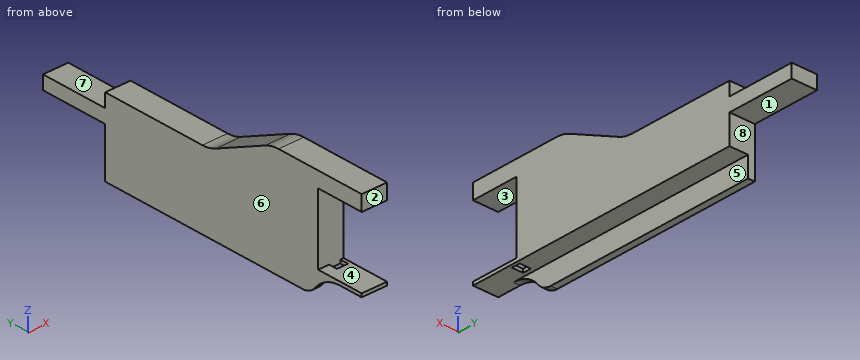
from build123d import *

# Parameters (mm, degrees)
EXTRUDE_1_DEPTH        = 26
EXTRUDE_2_DEPTH        = 19
FILLET_1_R             = 10
SKETCH_5_W             = 161
SKETCH_5_H             = 6
CUT_EXTRUDE_1_DEPTH    = 52
SKETCH_1_5_W           = 11
SKETCH_1_5_H           = 340
EXTRUDE_4_DEPTH        = 7
SKETCH_6_W             = 1.9
SKETCH_6_H             = 2
SKETCH_6_W_2           = 6.6
EXTRUDE_5_DEPTH        = 28
SKETCH_6_3_W           = 6.6
SKETCH_6_3_H           = 2
CUT_EXTRUDE_2_DEPTH    = 5
FILLET_2_R             = 20
SKETCH_6_4_W           = 15
SKETCH_6_4_H           = 10
SKETCH_6_4_H_2         = 9
EXTRUDE_6_DEPTH        = 30
SKETCH_6_5_W           = 15
SKETCH_6_5_H           = 9
EXTRUDE_7_DEPTH        = 28
EXTRUDE_8_DEPTH        = 15
FILLET_3_R             = 20
FILLET_3_OF_MIRROR_2_R = 20
FILLET_4_R             = 20
SKETCH_11_W            = 20
SKETCH_11_H            = 20
CUT_EXTRUDE_3_DEPTH    = 617
SKETCH_10_W            = 20
SKETCH_10_H            = 10
CUT_EXTRUDE_4_DEPTH    = 617
SKETCH_12_W            = 7.5
SKETCH_12_H            = 20
SKETCH_12_W_2          = 0.5
SKETCH_12_W_3          = 16.5
SKETCH_12_W_4          = 12
CUT_EXTRUDE_6_DEPTH    = 37


with BuildPart() as part:
    # 스케치1 → 보스-돌출1 (new body)
    with BuildSketch(Plane.XY):
        Polygon((-168, 0), (168, 0), (183, 0), (183, -340), (168, -340), (168, -20), (-168, -20), (-168, -340), (-183, -340), (-183, 0), align=None)
    extrude(amount=EXTRUDE_1_DEPTH)

    # 스케치1<4> → 보스-돌출2 (add)
    with BuildSketch(Plane.XY):
        Polygon((172, 0), (168, 0), (168, -20), (168, -340), (172, -340), align=None)
        Polygon((-168, -20), (-168, 0), (-172, 0), (-172, -340), (-168, -340), align=None)
    extrude(amount=-EXTRUDE_2_DEPTH)

    # 필렛1
    fillet_1_edges = [part.edges().sort_by_distance(p)[0] for p in [
        (170, 0, -19),
        (170, -340, -19),
        (-170, -340, -19),
        (-170, 0, -19),
    ]]
    fillet(fillet_1_edges, radius=FILLET_1_R)

    # 스케치5 → 컷-돌출1 (cut)
    with BuildSketch(Plane(origin=(0, 0, 0), x_dir=(1, 0, 0), z_dir=(0, 1, 0))):
        with Locations((-87.5, -3)):
            Rectangle(SKETCH_5_W, SKETCH_5_H)
        with Locations((87.5, -3)):
            Rectangle(SKETCH_5_W, SKETCH_5_H)
    extrude(amount=-CUT_EXTRUDE_1_DEPTH, mode=Mode.SUBTRACT)

    # 스케치1<5> → 보스-돌출4 (add)
    with BuildSketch(Plane.XY):
        with Locations((177.5, -170)):
            Rectangle(SKETCH_1_5_W, SKETCH_1_5_H)
        with Locations((-177.5, -170)):
            Rectangle(SKETCH_1_5_W, SKETCH_1_5_H)
    extrude(amount=-EXTRUDE_4_DEPTH)

    # 스케치6 → 보스-돌출5 (add)
    with BuildSketch(Plane.XZ.offset(340)):
        with Locations((-182.05, -6)):
            Rectangle(SKETCH_6_W, SKETCH_6_H)
        with Locations((-177.8, -6)):
            Rectangle(SKETCH_6_W_2, SKETCH_6_H)
        Polygon((-174.5, -7), (-172, -7), (-168, -7), (-168, -5), (-174.5, -5), align=None)
    extrude_5 = extrude(amount=EXTRUDE_5_DEPTH)

    # 스케치6<3> → 컷-돌출2 (cut)
    with BuildSketch(Plane.XZ.offset(340)):
        with Locations((-177.8, -6)):
            Rectangle(SKETCH_6_3_W, SKETCH_6_3_H)
    cut_extrude_2 = extrude(amount=CUT_EXTRUDE_2_DEPTH, mode=Mode.SUBTRACT)

    # 필렛2
    # the kernel refuses this fillet: 20 mm, written as the material it adds along each edge
    with BuildSketch(Plane(origin=(-172, -340, -7), x_dir=(0, -1, 0), z_dir=(1, 0, 0))) as fillet_2_piece_1:
        with BuildLine():
            CenterArc((14, 20), FILLET_2_R, 216.869897646, 53.130102354)
            Line((-2, 8), (-3.6, 6.8))
            ThreePointArc((-3.6, 6.8), (-2, 2), (-2, 0))
            Line((-2, 0), (0, -2))
            Line((0, -2), (14, -2))
            Line((14, -2), (14, 0))
        make_face()
    extrude(amount=4)

    # 스케치6<4> → 보스-돌출6 (add)
    with BuildSketch(Plane.XZ.offset(340)):
        with Locations((-175.5, 31)):
            Rectangle(SKETCH_6_4_W, SKETCH_6_4_H)
        with Locations((-175.5, 40.5)):
            Rectangle(SKETCH_6_4_W, SKETCH_6_4_H_2)
    extrude_6 = extrude(amount=-EXTRUDE_6_DEPTH)

    # 스케치6<5> → 보스-돌출7 (add)
    with BuildSketch(Plane.XZ.offset(340)):
        with Locations((-175.5, 40.5)):
            Rectangle(SKETCH_6_5_W, SKETCH_6_5_H)
    extrude_7 = extrude(amount=EXTRUDE_7_DEPTH)

    # 스케치9 → 보스-돌출8 (add)
    with BuildSketch(Plane.ZY.offset(183)):
        Polygon((26, -310), (45, -310), (26, -270), align=None)
    extrude_8 = extrude(amount=-EXTRUDE_8_DEPTH)

    # 필렛3
    fillet_3_edges = [part.edges().sort_by_distance(p)[0] for p in [
        (-175.5, -310, 45),
        (-175.5, -270, 26),
    ]]
    fillet(fillet_3_edges, radius=FILLET_3_R)

    # 대칭 복사2: 보스-돌출5, 컷-돌출2, 보스-돌출6, 보스-돌출7, 보스-돌출8 across plane
    add(extrude_5.mirror(Plane(origin=(0, 0, 0), x_dir=(0, 0, 1), z_dir=(1, 0, 0))))
    add(cut_extrude_2.mirror(Plane(origin=(0, 0, 0), x_dir=(0, 0, 1), z_dir=(1, 0, 0))), mode=Mode.SUBTRACT)
    add(extrude_6.mirror(Plane(origin=(0, 0, 0), x_dir=(0, 0, 1), z_dir=(1, 0, 0))))
    add(extrude_7.mirror(Plane(origin=(0, 0, 0), x_dir=(0, 0, 1), z_dir=(1, 0, 0))))
    add(extrude_8.mirror(Plane(origin=(0, 0, 0), x_dir=(0, 0, 1), z_dir=(1, 0, 0))))

    # 필렛3 of 대칭 복사2
    fillet_3_of_mirror_2_edges = [part.edges().sort_by_distance(p)[0] for p in [
        (175.5, -310, 45),
        (175.5, -270, 26),
    ]]
    fillet(fillet_3_of_mirror_2_edges, radius=FILLET_3_OF_MIRROR_2_R)

    # 필렛4
    # the kernel refuses this fillet: 20 mm, written as the material it adds along each edge
    with BuildSketch(Plane(origin=(172, -340, -7), x_dir=(0, 0.24253562503633938, -0.9701425001453302), z_dir=(-1, 0, 0))) as fillet_4_piece_1:
        with BuildLine():
            CenterArc((16.007351252, 18.432707503), FILLET_4_R, 194.036243468, 53.130102354)
            Line((-3.395498751, 13.581995002), (-5.335783751, 13.096923752))
            Line((-5.335783751, 13.096923752), (-1.940285, -0.48507125))
            Line((-1.940285, -0.48507125), (0.48507125, -1.940285))
            ThreePointArc((0.48507125, -1.940285), (2.42535625, -1.45521375), (7.470097251, -1.84327075))
            Line((7.470097251, -1.84327075), (8.246211251, 0))
        make_face()
    extrude(amount=4)

    # 스케치11 → 컷-돌출3 (cut)
    with BuildSketch(Plane.ZY.offset(-168)):
        with BuildLine():
            ThreePointArc((45, -314.508610159), (44.510394688, -310.110371974), (43.065550087, -305.927473868))
            Line((43.065550087, -305.927473868), (27.934449913, -274.072526132))
            ThreePointArc((27.934449913, -274.072526132), (26.489605312, -269.889628026), (26, -265.491389841))
            Line((26, -265.491389841), (26, -20))
            Line((26, -20), (6, -20))
            Line((6, -20), (6, 0))
            Line((6, 0), (-7, 0))
            Line((-7, 0), (-7, -354))
            Line((-7, -354), (-7, -368))
            Line((-7, -368), (-5, -368))
            Line((-5, -368), (-5, -340))
            Line((-5, -340), (36, -340))
            Line((36, -340), (36, -368))
            Line((36, -368), (45, -368))
            Line((45, -368), (45, -314.508610159))
        make_face()
        with Locations((16, -10)):
            Rectangle(SKETCH_11_W, SKETCH_11_H)
        with BuildLine():
            Line((-7, -354), (-7, 0))
            Line((-7, 0), (-9, 0))
            ThreePointArc((-9, 0), (-16.071067812, -2.928932188), (-19, -10))
            Line((-19, -10), (-19, -330))
            ThreePointArc((-19, -330), (-17.94427191, -334.472135955), (-15, -338))
            ThreePointArc((-15, -338), (-9.11145618, -345.05572809), (-7, -354))
        make_face()
    extrude(amount=CUT_EXTRUDE_3_DEPTH, mode=Mode.SUBTRACT)

    # 스케치10 → 컷-돌출4 (cut)
    with BuildSketch(Plane(origin=(183, 0, 0), x_dir=(0, 0, -1), z_dir=(1, 0, 0))):
        with Locations((-16, -15)):
            Rectangle(SKETCH_10_W, SKETCH_10_H)
    extrude(amount=-CUT_EXTRUDE_4_DEPTH, mode=Mode.SUBTRACT)

    # 스케치12 → 컷-돌출6 (cut)
    with BuildSketch(Plane.ZY.offset(-168)):
        Polygon((18.5, -162.5), (18.5, -183), (26, -183), (26, -20), (6, -20), (6, -10), (26, -10), (26, 0), (-7, 0), (-7, -183), (9.5, -183), (9.5, -162.5), align=None)
        with Locations((22.25, -193)):
            Rectangle(SKETCH_12_W, SKETCH_12_H)
        with Locations((18.25, -193)):
            Rectangle(SKETCH_12_W_2, SKETCH_12_H)
        with Locations((9.75, -193)):
            Rectangle(SKETCH_12_W_2, SKETCH_12_H)
        Polygon((18, -163), (18, -183), (18.5, -183), (18.5, -162.5), (9.5, -162.5), (9.5, -183), (10, -183), (10, -163), align=None)
        with Locations((1.25, -193)):
            Rectangle(SKETCH_12_W_3, SKETCH_12_H)
        with BuildLine():
            Line((-19, -183), (-7, -183))
            Line((-7, -183), (-7, 0))
            Line((-7, 0), (-9, 0))
            ThreePointArc((-9, 0), (-16.071067812, -2.928932188), (-19, -10))
            Line((-19, -10), (-19, -183))
        make_face()
        with Locations((-13, -193)):
            Rectangle(SKETCH_12_W_4, SKETCH_12_H)
    extrude(amount=-CUT_EXTRUDE_6_DEPTH, mode=Mode.SUBTRACT)


solid = part.part
Can you work these out from the model? Positions are in its coordinate system, mm. Face numbers are marked on the shaded views. A direction names the side the tool comes from. Coordinates: 2 decimals unless noted, no trailing zeros. Order: outer loops, then holes, each group sorted by start corner. A loop starts at its lowest first (then second) coordinate and runs counter-clockwise, first axis right, second up. Notation, with made-up numbers: (55.5, -38) -> (77.5, -38) arc R19 ccw to (77.5, -10) -> close; hole circle Ø9 at (2, -24.5). An arc over 180 degrees is marked (long way). Use one line per item in the form item = value.
Q1. We'd pull the mould along Z, two halves only. Please class the marked faces 1, 2, 3 and 4: released by +Z, released by -Z, zero draft, split by the parting line, or undercut.
From the geometry:
face_1 = released by -Z
face_2 = zero draft
face_3 = undercut
face_4 = undercut
Q2. Imagine slicing it at C-C, the plane y = -294. List the corners of the cut face in (x, z) for me, then the cut area to 3 significant figures.
From the geometry:
outline = (168, -19) -> (172, -19) -> (172, -7) -> (183, -7) -> (183, 37.4) -> (168, 37.4) -> close
area = 714 mm²
Q3. Which directions (+Z, -Z, +X, -X, +Y, -Y) give clear straight access to the entire face, cutting with the end or side of a thin tool? Please do the marked faces 5, 6, 7 and 8.
From the geometry:
face_5 = -Z, +X, +Y, -Y
face_6 = +Z, -Z, -X, +Y, -Y
face_7 = +Z, +X, -X, +Y
face_8 = -Z, +X, -X, +Y
Q4. I need wall thicknesses on L1, parallel to Y at x = 170, z = 5; L2, parallel to Y at x = 180.25, z = 12.5; L3, parallel to Z at x = 172.75, y = -181.5. Which ranges of each line are inside material? Lowest first, please.
From the geometry:
L1 = -340 to -203
L2 = -340 to -163
L3 = 10 to 18
Q5. Imagine slicing it at B-B, the plane y = -351. List the corners of the cut face in (x, z) for me.
From the geometry:
outline = (168, -7.23) -> (172, -7.23) -> (172, -7) -> (183, -7) -> (183, -5) -> (168, -5) -> close; (168, 36) -> (183, 36) -> (183, 45) -> (168, 45) -> close
Q6. Imagine slicing it at A-A, the plane x = 177. List the corners of the cut face in (y, z) for me, then the cut area to 3 significant figures.
From the geometry:
outline = (-368, -7) -> (-345, -7) -> (-345, -5) -> (-368, -5) -> close; (-368, 36) -> (-340, 36) -> (-340, -7) -> (-203, -7) -> (-203, 10) -> (-163, 10) -> (-163, 18) -> (-203, 18) -> (-203, 26) -> (-265.49, 26) arc R20 cw to (-274.07, 27.93) -> (-305.93, 43.07) arc R20 ccw to (-314.51, 45) -> (-368, 45) -> close
area = 6,090 mm²
Q7. Will these pins go through, and if not, where does the flat tip stop? P1, Ø4.5, axis at x = 174, y = -186, coming from the +Z side; P2, Ø5, axis at x = 171, z = 22.5, coming from the +Y side; P3, Ø4.5, axis at x = 174, y = -186.5, coming from the -Z side.
From the geometry:
P1 = 18
P2 = -203
P3 = 10
Q8. Imagine slicing it at D-D, the plane z = 2. List the corners of the cut face in (x, y) for me, then the cut area to 4 significant figures.
From the geometry:
outline = (168, -340) -> (183, -340) -> (183, -203) -> (168, -203) -> close
area = 2,055 mm²
